```python
from build123d import *

# Parameters (mm, degrees)
BOSS_EXTRUDE1_DEPTH = 1.9


with BuildPart() as part:
    # Sketch1 → Boss-Extrude1 (new body)
    with BuildSketch(Plane(origin=(0, 0, 0), x_dir=(1, 0, 0), z_dir=(0, 1, 0))):
        Polygon((2.875222959, -7.101510951), (7.054616202, -2.988436898), (7.101510951, 2.875222959), (2.988436898, 7.054616202), (-2.875222959, 7.101510951), (-7.054616202, 2.988436898), (-7.101510951, -2.875222959), (-2.988436898, -7.054616202), align=None)
        with BuildLine():
            Line((-4.854615023, 0.9), (-4.037336024, 0.9))
            Line((-4.037336024, 0.9), (-4.037336024, -0.9))
            Line((-4.037336024, -0.9), (-4.854615023, -0.9))
            ThreePointArc((-4.854615023, -0.9), (0, -4.937336024), (4.854615023, -0.9))
            Line((4.854615023, -0.9), (4.037336024, -0.9))
            Line((4.037336024, -0.9), (4.037336024, 0.9))
            Line((4.037336024, 0.9), (4.854615023, 0.9))
            ThreePointArc((4.854615023, 0.9), (0, 4.937336024), (-4.854615023, 0.9))
        make_face(mode=Mode.SUBTRACT)
    extrude(amount=BOSS_EXTRUDE1_DEPTH)


solid = part.part
```
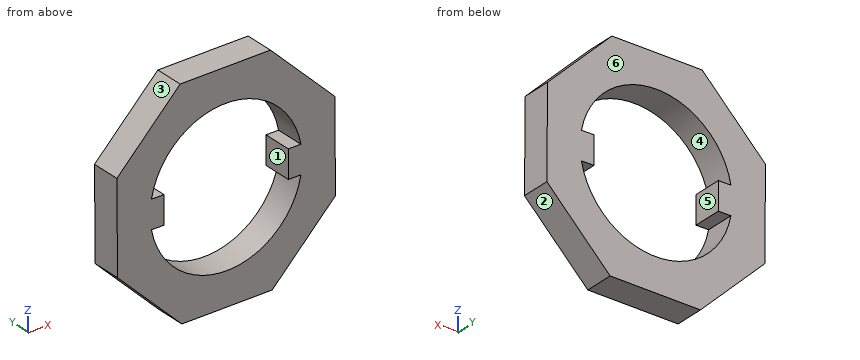
Check sheet for the modelled part. Datum: model origin and axes. Units: mm. Face numbers are marked on the shaded views. A direction names the side the tool comes from. Round coordinates to 2 decimals unless told otherwise and drop trailing zeros. Order: outer loops, then holes, each group sorted by start corner. A loop starts at its lowest first (then second) coordinate and runs counter-clockwise, first axis right, second up. Notation, with made-up numbers: (59, -36) -> (99, -36) arc R31 cw to (99, 2) -> close; hole circle Ø2 at (-39, 18.25). An arc over 180 degrees is marked (long way). One line per item, written item: value. Start each with the question number.
Q1. Gauge pin test, flat ends, axial feed: pin 1 Ø0.9 at (x, y) = (4.5, 0.5) entering from -Z; pin 2 Ø1 at (x, y) = (-3.5, 1) entering from -Z; pin 3 Ø0.9 at (x, y) = (4.5, 1) entering from +Z. Record the tip position at first contact, or that the pin passes through.
Q2. Cross-section at B-B (x = -1). Record the boundary of the cut face in (y, z) (3 decimals).
Q3. Cross-section at A-A (y = 0.7). Record the boundary of the cut face in (x, z).
Q4. Mould release check, pull along Z, two halves, no side actions. Record for the marked faces 3, 4, 5 and 6: pulls with the +Z half, pulls with the -Z half, needs draft (parallel to the pull), parting line crosses it, or undercut.
Q5. Cross-section at D-D (z = 5.25). Record the boundary of the cut face in (x, y), and give its area (3 significant figures).
Q6. Thickness scan on line 1 (Z direction, x = -4.5, y = 1.85); line 2 (X direction, y = 1.6, z = -4.25); line 3 (X direction, y = 0.75, z = -4). Record the ranges inside material, lowest first.
Q7. Set-up check for the marked faces 1 and 2: record each of +Z, -Z, +X, -X, +Y, -Y from which the full face is reachable in a straight line by a thin tool's end or side.
Q8. Cross-section at C-C (z = -2.5). Record the boundary of the cut face in (x, y), and give its area (3 significant figures).
Completed:
1. pin 1: stops at z = -5.98
1. pin 2: stops at z = -6.98
1. pin 3: stops at z = 5.95
2. outline: (0, -7.087) -> (1.9, -7.087) -> (1.9, -4.835) -> (0, -4.835) -> close; (0, 4.835) -> (1.9, 4.835) -> (1.9, 7.071) -> (0, 7.071) -> close
3. outline: (-7.1, 2.88) -> (-7.05, -2.99) -> (-2.88, -7.1) -> (2.99, -7.05) -> (7.1, -2.88) -> (7.05, 2.99) -> (2.88, 7.1) -> (-2.99, 7.05) -> close; hole (-4.85, -0.9) arc R4.94 ccw to (4.85, -0.9) -> (4.04, -0.9) -> (4.04, 0.9) -> (4.85, 0.9) arc R4.94 ccw to (-4.85, 0.9) -> (-4.04, 0.9) -> (-4.04, -0.9) -> close
4. face 3: pulls with the +Z half
4. face 4: undercut
4. face 5: undercut
4. face 6: needs draft
5. outline: (-4.76, 0) -> (4.76, 0) -> (4.76, 1.9) -> (-4.76, 1.9) -> close
5. area: 18.1 mm²
6. line 1: z = -5.5 to -2.03, -0.9 to 0.9, 2.03 to 5.52
6. line 2: x = -5.77 to -2.51, 2.51 to 5.75
6. line 3: x = -6.03 to -2.89, 2.89 to 5.99
7. face 1: +Y, -Y
7. face 2: -Z, +X, +Y, -Y
8. outline: (-7.06, 0) -> (-4.26, 0) -> (-4.26, 1.9) -> (-7.06, 1.9) -> close; (4.26, 0) -> (7.1, 0) -> (7.1, 1.9) -> (4.26, 1.9) -> close
8. area: 10.7 mm²
